Read the model definition and answer for the solid it produces. Units are mm, in the model's axes. A direction names the side the tool comes from. Give positions to 0.01 mm unless a question says otherwise; leave off trailing zeros. Loops run counter-clockwise (first coordinate to the right, second up) from the corner with the lowest first, then second, coordinate; pieces in that order, holes last. Notation, with made-up numbers: (65.25, 72.25) - (76.25, 72.25) arc R19 ccw to (76.25, 79.25) - close; hole circle Ø11 at (18.5, 12). An arc over 180 degrees is marked (long way). Write item = value, one per line. Start each with the question number.
Autodesk Inventor part; units mm, degrees
ref_plane "Pracovní rovina1" through (0, 0, 0) normal (0, 0, -1) x (-1, 0, 0)
ref_plane "YZ Plane" through (0, 0, 0) normal (1, 0, 0) x (0, 1, 0)
ref_plane "XZ Plane" through (0, 0, 0) normal (0, 1, 0) x (-1, 0, 0)
sketch "Náčrt1" plane through (0, 0, 0) normal (0, 0, 1) x (1, 0, 0)
  line L0 (-95, 0) -> (80, 0)
  line L1 (0, -73.5) -> (0, 73.5)
  line L2 (-55, 52.5) -> (55, 52.5)
  line L3 (55, 52.5) -> (55, 22.5)
  line L4 (55, 22.5) -> (-55, 22.5)
  line L5 (-55, 22.5) -> (-55, 52.5)
  line L6 (40, -52.5) -> (10, -52.5)
  line L7 (10, -52.5) -> (10, 22.5)
  line L8 (10, 22.5) -> (40, 22.5)
  line L9 (40, 22.5) -> (40, -52.5)
  circle A0 centre (-55, 37.5) radius 15
  point P0 (0, 0)
  dimension "d0" = 30
  dimension "d1" = 110
  dimension "d2" = 30
  dimension "d3" = 15
  dimension "d4" = 75
extrude "Vysunutí1" add sketch "Náčrt1" along normal blind 14 contours L7 L4 L9 L0 | L0 L9 L6 L7 | L4 A0 L2 L1 | L1 L2 L3 L4 | A0 L5 | L5 A0
sketch "Náčrt2" plane through (0, 0, 0) normal (0, 0, -1) x (-1, 0, 0)
  line L0 (-55, 52.5) -> (55, 52.5)
  line L1 (-55, 52.5) -> (55, 52.5)
  line L2 (-55, 22.5) -> (-55, 52.5)
  line L3 (-40, 22.5) -> (-55, 22.5)
  line L4 (-40, -52.5) -> (-40, 22.5)
  line L5 (-10, -52.5) -> (-40, -52.5)
  line L6 (-10, 22.5) -> (-10, -52.5)
  line L7 (55, 22.5) -> (-10, 22.5)
  arc A0 (55, 22.5) -> (55, 52.5) centre (55, 37.5) ccw
  point P0 (0, 0)
hole "Díra1" at (-55, 37.5, 0) direction (0, 0, 1) diameter 12 end through all counterbore diameter 20 counterbore depth 7
chamfer "Zkosení1" distance 3 angle 45 8 edges at (0, 52.5, 14) (-70, 37.5, 14) (-22.5, 22.5, 14) (10, -15, 14) (40, -15, 14) (47.5, 22.5, 14) (55, 37.5, 14) (25, -52.5, 14)
sketch "Náčrt3" plane through (0, 0, 14) normal (0, 0, 1) x (1, 0, 0)
  circle A0 centre (-55, 37.5) radius 6
  line L0 (-55, 49.5) -> (52, 49.5)
  arc A1 (-55, 49.5) -> (-55, 25.5) centre (-55, 37.5) ccw
  line L1 (13, 25.5) -> (-55, 25.5)
  line L2 (13, -49.5) -> (13, 25.5)
  line L3 (37, -49.5) -> (13, -49.5)
  line L4 (37, 25.5) -> (37, -49.5)
  line L5 (52, 25.5) -> (37, 25.5)
  line L6 (52, 49.5) -> (52, 25.5)
  line L7 (0, 73.5) -> (0, -73.5)
  line L8 (-95, 0) -> (80, 0)
  point P0 (0, 0)
  point P1 (35, 37.5)
  dimension "d17" = 12
  dimension "d18" = 17
hole "Díra2" at (35, 37.5, 14) direction (0, 0, -1) diameter 6.5 end through all counterbore diameter 11 counterbore depth 4
pattern_linear "Obdélníkové pole1" count 2 spacing 20 along (-1, 0, 0) of "Díra2"
sketch "Náčrt4" plane through (0, 0, 14) normal (0, 0, 1) x (1, 0, 0)
  line L0 (-95, 0) -> (80, 0)
  line L1 (0, -73.5) -> (0, 73.5)
  circle A0 centre (15, 37.5) radius 5.5
  circle A1 centre (35, 37.5) radius 5.5
  circle A2 centre (-55, 37.5) radius 6
  line L2 (-55, 49.5) -> (52, 49.5)
  arc A3 (-55, 49.5) -> (-55, 25.5) centre (-55, 37.5) ccw
  line L3 (13, 25.5) -> (-55, 25.5)
  line L4 (13, -49.5) -> (13, 25.5)
  line L5 (37, -49.5) -> (13, -49.5)
  line L6 (37, 25.5) -> (37, -49.5)
  line L7 (52, 25.5) -> (37, 25.5)
  line L8 (52, 49.5) -> (52, 25.5)
  line L9 (-33.7624, 29.5) -> (-28.7624, 29.5)
  line L10 (-28.7624, 29.5) -> (-38, 45.5)
  line L11 (-28.7624, 29.5) -> (-10.2872, 29.5) construction
  line L12 (-33.7624, 29.5) -> (-43, 45.5)
  line L13 (-43, 45.5) -> (-38, 45.5)
  point P0 (0, 0)
  dimension "d29" = 120
  dimension "d31" = 5
  dimension "d32" = 4
  dimension "d33" = 4
  dimension "d34" = 12
extrude "Vysunutí2" cut sketch "Náčrt4" against normal through all contours L12 L13 L10 L9
chamfer "Zkosení2" distance 1 angle 45 4 edges at (-38.3812, 37.5, 14) (-40.5, 45.5, 14) (-33.3812, 37.5, 14) (-31.2624, 29.5, 14)
pattern_linear "Obdélníkové pole2" count 3 spacing 12 along (1, 0, 0) of "Vysunutí2", "Zkosení2"
sketch "Náčrt5" plane through (0, 0, 14) normal (0, 0, 1) x (1, 0, 0)
  line L0 (-32.7321, 46.5) -> (-22.3397, 28.5)
  line L1 (-25.4226, 46.5) -> (-32.7321, 46.5)
  line L2 (-15.0303, 28.5) -> (-25.4226, 46.5)
  line L3 (-22.3397, 28.5) -> (-15.0303, 28.5)
  line L4 (-55, 49.5) -> (52, 49.5)
  arc A0 (-55, 49.5) -> (-55, 25.5) centre (-55, 37.5) ccw
  line L5 (13, 25.5) -> (-55, 25.5)
  line L6 (13, -49.5) -> (13, 25.5)
  line L7 (37, -49.5) -> (13, -49.5)
  line L8 (37, 25.5) -> (37, -49.5)
  line L9 (52, 25.5) -> (37, 25.5)
  line L10 (52, 49.5) -> (52, 25.5)
  circle A1 centre (-55, 37.5) radius 6
  circle A2 centre (35, 37.5) radius 5.5
  circle A3 centre (15, 37.5) radius 5.5
  line L11 (-27.0303, 28.5) -> (-37.4226, 46.5)
  line L12 (-34.3397, 28.5) -> (-27.0303, 28.5)
  line L13 (-44.7321, 46.5) -> (-34.3397, 28.5)
  line L14 (-37.4226, 46.5) -> (-44.7321, 46.5)
  line L15 (-20.7321, 46.5) -> (-10.3397, 28.5)
  line L16 (-13.4226, 46.5) -> (-20.7321, 46.5)
  line L17 (-3.0303, 28.5) -> (-13.4226, 46.5)
  line L18 (-10.3397, 28.5) -> (-3.0303, 28.5)
  line L19 (0, -73.5) -> (0, 73.5)
  line L20 (27, 19.9641) -> (29, 16.5)
  line L21 (29, 16.5) -> (27, 13.0359)
  line L22 (27, 13.0359) -> (23, 13.0359)
  line L23 (23, 13.0359) -> (21, 16.5)
  line L24 (21, 16.5) -> (23, 19.9641)
  line L25 (23, 19.9641) -> (27, 19.9641)
  point P0 (0, 0)
  point P1 (25, 16.5)
  dimension "d43" = 4
  dimension "d44" = 9
  dimension "d45" = 12
  dimension "d52" = 3.4641
extrude "Vysunutí3" cut sketch "Náčrt5" against normal through all contours L20 L21 L22 L23 L24 L25
chamfer "Zkosení3" distance 1 angle 45 6 edges at (25, 19.9641, 14) (28, 18.2321, 14) (28, 14.7679, 14) (25, 13.0359, 14) (22, 14.7679, 14) (22, 18.2321, 14)
pattern_linear "Obdélníkové pole3" count 4 spacing 18 along (0, -1, 0) of "Vysunutí3", "Zkosení3"
ref_plane "Pracovní rovina1" through (0, 0, 0) normal (0, 0, -1) x (-1, 0, 0)
sketch "Náčrt7" plane through (0, 0, 0) normal (0, 0, -1) x (-1, 0, 0)
  line L0 (-29, -37.5) -> (-27, -34.0359)
  line L1 (-27, -34.0359) -> (-23, -34.0359)
  line L2 (-23, -34.0359) -> (-21, -37.5)
  line L3 (-21, -37.5) -> (-23, -40.9641)
  line L4 (-23, -40.9641) -> (-27, -40.9641)
  line L5 (-27, -40.9641) -> (-29, -37.5)
  line L6 (-29, -19.5) -> (-27, -16.0359)
  line L7 (-27, -16.0359) -> (-23, -16.0359)
  line L8 (-23, -16.0359) -> (-21, -19.5)
  line L9 (-21, -19.5) -> (-23, -22.9641)
  line L10 (-23, -22.9641) -> (-27, -22.9641)
  line L11 (-27, -22.9641) -> (-29, -19.5)
  line L12 (-29, -1.5) -> (-27, 1.9641)
  line L13 (-27, 1.9641) -> (-23, 1.9641)
  line L14 (-23, 1.9641) -> (-21, -1.5)
  line L15 (-21, -1.5) -> (-23, -4.9641)
  line L16 (-23, -4.9641) -> (-27, -4.9641)
  line L17 (-27, -4.9641) -> (-29, -1.5)
  line L18 (-21, 16.5) -> (-23, 13.0359)
  line L19 (-23, 13.0359) -> (-27, 13.0359)
  line L20 (-27, 13.0359) -> (-29, 16.5)
  line L21 (-29, 16.5) -> (-27, 19.9641)
  line L22 (-27, 19.9641) -> (-23, 19.9641)
  line L23 (-23, 19.9641) -> (-21, 16.5)
  line L24 (19, 45.5) -> (9.7624, 29.5)
  line L25 (9.7624, 29.5) -> (4.7624, 29.5)
  line L26 (4.7624, 29.5) -> (14, 45.5)
  line L27 (14, 45.5) -> (19, 45.5)
  line L28 (31, 45.5) -> (21.7624, 29.5)
  line L29 (21.7624, 29.5) -> (16.7624, 29.5)
  line L30 (16.7624, 29.5) -> (26, 45.5)
  line L31 (26, 45.5) -> (31, 45.5)
  line L32 (28.7624, 29.5) -> (38, 45.5)
  line L33 (38, 45.5) -> (43, 45.5)
  line L34 (43, 45.5) -> (33.7624, 29.5)
  line L35 (33.7624, 29.5) -> (28.7624, 29.5)
  circle A0 centre (-15, 37.5) radius 3.25
  circle A1 centre (-35, 37.5) radius 3.25
  circle A2 centre (55, 37.5) radius 10
  line L36 (-55, 52.5) -> (55, 52.5)
  line L37 (-55, 22.5) -> (-55, 52.5)
  line L38 (-40, 22.5) -> (-55, 22.5)
  line L39 (-40, -52.5) -> (-40, 22.5)
  line L40 (-10, -52.5) -> (-40, -52.5)
  line L41 (-10, 22.5) -> (-10, -52.5)
  line L42 (55, 22.5) -> (-10, 22.5)
  arc A3 (55, 22.5) -> (55, 52.5) centre (55, 37.5) ccw
  line L43 (-40, 13.8397) -> (-55, 22.5)
  line L44 (-10, 13.8397) -> (5, 22.5)
  line L45 (-10, 22.5) -> (-10, -52.5)
  line L46 (-10, 13.8397) -> (-10, 22.5)
  line L47 (-10, 22.5) -> (5, 22.5)
  line L48 (-40, -52.5) -> (-40, 22.5)
  line L49 (-40, 13.8397) -> (-40, 22.5)
  line L50 (-40, 22.5) -> (-55, 22.5)
  point P0 (0, 0)
  dimension "d68" = 15
  dimension "d69" = 15
  dimension "d70" = 30
  dimension "d71" = 30
extrude "Vysunutí4" add sketch "Náčrt7" against normal blind 11 contours L38 L39 L43 | L44 L41 L42
properties part number "blet_leg_30x30_3D tisk"
1. A cutting plane is placed at A-A on x = 15. Give the vertices of the cut face in (y, z).
2. A cutting plane is placed at B-B on y = -8. Give the vertices of the cut face in (x, z), and give its area (3 significant figures).
3. Consider line 1 along Y through (x, z) = (15, 4.75); line 2 along Y through (x, z) = (-55, 9); line 3 along X through (y, z) = (33, 4.5). Determine where each line is inside the solid, lowest interval first. Write a range as [from, to].
4. A tool of negligible diameter and unlimited length cuts with its end or side. For faces 5 (the flat face through (2.6, 18.11, 5.42)), 6 (the flat face through (21.56, -3.45, 13.49)), 7 (the flat face through (22.014, -39.256, 6.591)), from which of +Z, -Z, +X, -X, +Y, -Y can it reach the whole face along a straight path? Write none if from no direction.
5. A cutting plane is placed at C-C on z = 2.5. Give the number of separate pieces and of enclosed holes in the cut face, and give its area (3 significant figures).
6. Given P1, Ø3, axis at y = -25.5, z = 3.5, coming from the +X side; P2, Ø7, axis at x = 47.5, y = 20, coming from the +Z side; P3, Ø4, axis at x = -15.5, z = 6.5, coming from the -Y side, each flat-ended and moving along its own axis, determine where each tip first touches the part or whether it passes through.
7. For a pull along X with two mould halves and no side action, classify faces 1 (the cylindrical face through (-69.996, 37.17, 5.423)), 2 (the flat face through (19, 38, 10)), 3 (the flat face through (-33.32, 37.39, 6.59)), 4 (the flat face through (-30, 22.5, 5)) as released by +X, released by -X, zero draft, split by the parting line, or undercut.
Reply:
q1.outline = (-52.5, 0) - (34.25, 0) - (34.25, 10) - (32, 10) - (32, 14) - (-49.5, 14) - (-52.5, 11) - close; (40.75, 0) - (52.5, 0) - (52.5, 11) - (49.5, 14) - (43, 14) - (43, 10) - (40.75, 10) - close
q2.outline = (10, 0) - (40, 0) - (40, 11) - (37, 14) - (13, 14) - (10, 11) - close
q2.area = 411 mm^2
q3.line_1 = [-52.5, 34.25], [40.75, 52.5]
q3.line_2 = [22.5, 31.5], [43.5, 52.5]
q3.line_3 = [-69.31, -63.93], [-46.07, -35.78], [-30.78, -23.78], [-18.78, -11.78], [-6.78, 55]
q4.face_5 = +Z, -Z, -X, -Y
q4.face_6 = +Z
q4.face_7 = +Z, -Z
q5.separate_pieces = 1
q5.enclosed_holes = 10
q5.area = 5,250 mm^2
q6.P1 = 40
q6.P2 = 12
q6.P3 = 22.5
q7.face_1 = released by -X
q7.face_2 = undercut
q7.face_3 = undercut
q7.face_4 = zero draft
